```python
from build123d import *

# Parameters (mm, degrees)
BOSS_EXTRUDE1_DEPTH     = 5
CUT_EXTRUDE1_DEPTH      = 9.189780217
CUT_EXTRUDE1_DEPTH_BACK = 9.189780217
SKETCH2_R               = 2.5
FILLET1_R               = 0.25
FILLET2_R               = 0.25


with BuildPart() as part:
    # Sketch1 → Boss-Extrude1 (new, symmetric)
    with BuildSketch(Plane.XY):
        Polygon((-2.9, -0.75), (-2.9, 0.75), (2.9, 0.75), (2.9, -0.75), (4.9, -0.75), (4.9, -2.25), (2.9, -4.25), (-2.9, -4.25), (-4.9, -2.25), (-4.9, -0.75), align=None)
    extrude(amount=BOSS_EXTRUDE1_DEPTH, both=True)

    # Sketch2 → Cut-Extrude1 (cut, two sides: drawn at the far end of the back side and taken through both)
    with BuildSketch(Plane(origin=(0, 0, 0), x_dir=(1, 0, 0), z_dir=(0, 1, 0)).offset(-CUT_EXTRUDE1_DEPTH_BACK)):
        with Locations(Location((0, 0, 0), (0, 0, 270))):
            Circle(SKETCH2_R)
    extrude(amount=CUT_EXTRUDE1_DEPTH + CUT_EXTRUDE1_DEPTH_BACK, mode=Mode.SUBTRACT)

    # Fillet1
    fillet1_edges = [part.edges().sort_by_distance(p)[0] for p in [
        (2.9, -0.75, 0),
        (4.9, -2.25, 0),
        (-4.9, -2.25, 0),
        (-2.9, -0.75, 0),
    ]]
    fillet(fillet1_edges, radius=FILLET1_R)

    # Fillet2
    fillet2_edges = [part.edges().sort_by_distance(p)[0] for p in [
        (0, -4.25, -2.5),
        (0, 0.75, -2.5),
    ]]
    fillet(fillet2_edges, radius=FILLET2_R)


solid = part.part
```
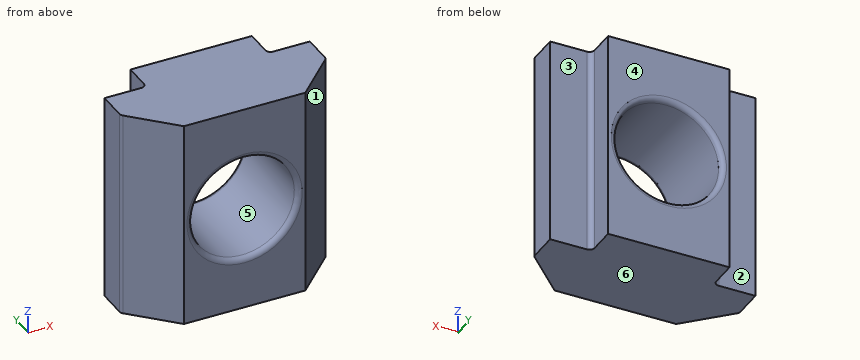
Work out the finished part from the listing and answer in its coordinate system (mm). Face numbers are marked on the shaded views. A direction names the side the tool comes from. Give positions to 0.01 mm unless a question says otherwise; leave off trailing zeros. Order: outer loops, then holes, each group sorted by start corner. A loop starts at its lowest first (then second) coordinate and runs counter-clockwise, first axis right, second up. Notation, with made-up numbers: (32, 74) - (86, 74) arc R25 ccw to (86, 109) - close; hole circle Ø6 at (56, -26.75). An arc over 180 degrees is marked (long way). One line per item, written item: value. Start each with the question number.
1. Section A-A, the plane z = 0 is taken. Write down the section's boundary in (x, y), then the cut area to 3 significant figures.
2. Consider line 1 (Z direction, x = 0, y = -3.2); line 2 (X direction, y = -1.3, z = 0); line 3 (X direction, y = -1.2, z = 0.5). Determine where each line is inside the solid, lowest interval first.
3. For a pull along Z with two mould halves and no side action, classify the marked faces 4, 5 and 6 as released by +Z, released by -Z, zero draft, split by the parting line, or undercut.
4. Which of the six approach directions +Z, -Z, +X, -X, +Y, -Y give full straight-line access (tool end or side, diameter ignored) to the marked faces 1, 2 and 3?
5. Section D-D, the plane z = 4 is taken. Write down the section's boundary in (x, y).
6. Each of these flat-tipped pins is pushed along its axis until it touches: pin 1 Ø1.9 at (x, z) = (-4.5, 1) entering from +Y; pin 2 Ø5 at (x, z) = (-2, 0) entering from +Y. Where does it stop, or does it pass through?
7. Section B-B, the plane y = -3.1 is taken. Write down the section's boundary in (x, z).
8. Section C-C, the plane x = 0 is taken. Write down the section's boundary in (y, z).
Filled sheet:
1. outline: (-4.9, -2.15) arc R0.25 ccw to (-4.83, -2.32) - (-2.9, -4.25) - (-2.75, -4.25) arc R0.25 ccw to (-2.5, -4) - (-2.5, 0.5) arc R0.25 ccw to (-2.75, 0.75) - (-2.9, 0.75) - (-2.9, -0.5) arc R0.25 cw to (-3.15, -0.75) - (-4.9, -0.75) - close; (2.5, -4) arc R0.25 ccw to (2.75, -4.25) - (2.9, -4.25) - (4.83, -2.32) arc R0.25 ccw to (4.9, -2.15) - (4.9, -0.75) - (3.15, -0.75) arc R0.25 cw to (2.9, -0.5) - (2.9, 0.75) - (2.75, 0.75) arc R0.25 ccw to (2.5, 0.5) - close
1. area: 14.0 mm²
2. line 1: -5 to -2.5, 2.5 to 5
2. line 2: -4.9 to -2.5, 2.5 to 4.9
2. line 3: -4.9 to -2.45, 2.45 to 4.9
3. face 4: zero draft
3. face 5: undercut
3. face 6: released by -Z
4. face 1: +Z, -Z, +X, -Y
4. face 2: +Z, -Z, -X, +Y
4. face 3: +Z, -Z, +X, +Y
5. outline: (-4.9, -2.15) arc R0.25 ccw to (-4.83, -2.32) - (-2.9, -4.25) - (2.9, -4.25) - (4.83, -2.32) arc R0.25 ccw to (4.9, -2.15) - (4.9, -0.75) - (3.15, -0.75) arc R0.25 cw to (2.9, -0.5) - (2.9, 0.75) - (-2.9, 0.75) - (-2.9, -0.5) arc R0.25 cw to (-3.15, -0.75) - (-4.9, -0.75) - close
6. pin 1: y = -0.75
6. pin 2: y = 0.75
7. outline: (-4.05, -5) - (4.05, -5) - (4.05, 5) - (-4.05, 5) - close; hole circle Ø5 at (0, 0)
8. outline: (-4.25, -5) - (0.75, -5) - (0.75, -2.75) arc R0.25 ccw to (0.5, -2.5) - (-4, -2.5) arc R0.25 ccw to (-4.25, -2.75) - close; (-4.25, 2.75) arc R0.25 ccw to (-4, 2.5) - (0.5, 2.5) arc R0.25 ccw to (0.75, 2.75) - (0.75, 5) - (-4.25, 5) - close
